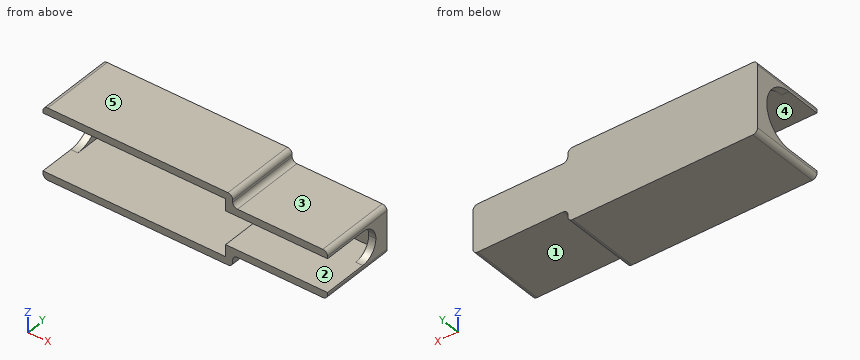
from build123d import *

# Parameters (mm, degrees)
F1_DEPTH = 16
F2_T     = -1.5
F4_DEPTH = 25
F6_DEPTH = 25
F7_R     = 1


with BuildPart() as f1:
    # F0 (on Front) → F1 (new body)
    with BuildSketch(Plane.XZ):
        Polygon((10, 7.5), (-30, 7.5), (-30, -7.5), (10, -7.5), (10, -5), (30, -5), (30, 5), (10, 5), align=None)
    extrude(amount=F1_DEPTH)

    # F2
    f2_openings = [f1.faces().sort_by_distance(p)[0] for p in [
        (-2.5, -16, 0),
    ]]
    offset(amount=F2_T, openings=f2_openings, kind=Kind.INTERSECTION)

    # F3 (on face) → F4 (cut)
    with BuildSketch(Plane.YZ.offset(30)):
        with BuildLine():
            ThreePointArc((-6.5, -3.5), (-10, 0), (-6.5, 3.5))
            Line((-6.5, 3.5), (-16, 3.5))
            Line((-16, 3.5), (-16, -3.5))
            Line((-16, -3.5), (-6.5, -3.5))
        make_face()
        with BuildLine():
            ThreePointArc((-6.5, -3.5), (-4.0251262658, -2.4748737342), (-3, 0))
            ThreePointArc((-3, 0), (-4.0251262658, 2.4748737342), (-6.5, 3.5))
            ThreePointArc((-6.5, 3.5), (-10, 0), (-6.5, -3.5))
        make_face()
    extrude(amount=-F4_DEPTH, mode=Mode.SUBTRACT)

    # F5 (on face) → F6 (cut)
    with BuildSketch(Plane(origin=(-30, 0, 0), x_dir=(0, -1, 0), z_dir=(-1, 0, 0))):
        with BuildLine():
            ThreePointArc((8.5, -6), (12.7426406871, -4.2426406871), (14.5, 0))
            ThreePointArc((14.5, 0), (12.7426406871, 4.2426406871), (8.5, 6))
            ThreePointArc((8.5, 6), (2.5, 0), (8.5, -6))
        make_face()
        with BuildLine():
            ThreePointArc((8.5, 6), (12.7426406871, 4.2426406871), (14.5, 0))
            ThreePointArc((14.5, 0), (12.7426406871, -4.2426406871), (8.5, -6))
            Line((8.5, -6), (16, -6))
            Line((16, -6), (16, 6))
            Line((16, 6), (8.5, 6))
        make_face()
    extrude(amount=-F6_DEPTH, mode=Mode.SUBTRACT)

    # F7
    f7_edges = [f1.edges().sort_by_distance(p)[0] for p in [
        (-30, -8, -7.5),
        (-30, -8, 7.5),
        (10, -8, 5),
        (10, -8, 7.5),
        (10, -8, -7.5),
        (10, -8, -5),
        (30, -8, -5),
        (30, -8, 5),
    ]]
    fillet(f7_edges, radius=F7_R)


solid = f1.part
The model under review builds one solid part; all positions refer to its coordinate system, in mm. Face numbers are marked on the shaded views. A direction names the side the tool comes from. Coordinates: 2 decimals unless noted, no trailing zeros. Order: outer loops, then holes, each group sorted by start corner. A loop starts at its lowest first (then second) coordinate and runs counter-clockwise, first axis right, second up. Notation, with made-up numbers: (7.5, 79.25) -> (50.5, 79.25) arc R22 ccw to (50.5, 115.25) -> close; hole circle Ø10 at (81.5, 3.25). An arc over 180 degrees is marked (long way). Answer in a Markdown table with one row per item.
(1) Consider section B-B (x = -18). Write out the cut boundary in (y, z), plus the area to 3 significant figures.
Answers:
| item | result |
|---|---|
| outline | (-16, -7.5) -> (0, -7.5) -> (0, 7.5) -> (-16, 7.5) -> (-16, 6) -> (-1.5, 6) -> (-1.5, -6) -> (-16, -6) -> close |
| area | 66.0 mm² |
(2) Wall thickness on line 1 along Z through (x, y) = (-11, -9); line 2 along Z through (x, y) = (13, -11.75); line 3 along Y through (x, z) = (-16, 2.25): over which ranges is each line inside the solid? List them lowest first.
Answers:
| item | result |
|---|---|
| line 1 | -7.5 to -6, 6 to 7.5 |
| line 2 | -5 to -3.5, 3.5 to 5 |
| line 3 | -1.5 to 0 |
(3) Consider section D-D (x = 19). Write out the cut boundary in (y, z).
Answers:
| item | result |
|---|---|
| outline | (-16, -5) -> (0, -5) -> (0, 5) -> (-16, 5) -> (-16, 3.5) -> (-1.5, 3.5) -> (-1.5, -3.5) -> (-16, -3.5) -> close |
(4) Machinability: for the marked faces 4 and 5, which of the approach directions +Z, -Z, +X, -X, +Y, -Y give a long, thin tool a straight path to every point of the face, cutting with its end or side? Answer none if there is none.
Answers:
| item | result |
|---|---|
| face 4 | -Y |
| face 5 | +Z, +X, -X, +Y, -Y |
(5) Consider section A-A (y = -11.5). Write out the cut boundary in (x, z), plus the area to 3 significant figures.
Answers:
| item | result |
|---|---|
| outline | (-30, -6.5) arc R1 ccw to (-29, -7.5) -> (9, -7.5) arc R1 ccw to (10, -6.5) -> (10, -6) arc R1 cw to (11, -5) -> (29, -5) arc R1 ccw to (30, -4) -> (30, -3.5) -> (8.5, -3.5) -> (8.5, -6) -> (-30, -6) -> close; (-30, 6) -> (8.5, 6) -> (8.5, 3.5) -> (30, 3.5) -> (30, 4) arc R1 ccw to (29, 5) -> (11, 5) arc R1 cw to (10, 6) -> (10, 6.5) arc R1 ccw to (9, 7.5) -> (-29, 7.5) arc R1 ccw to (-30, 6.5) -> close |
| area | 187 mm² |
(6) Insertion check: pin 1 (3 mm diameter, centred on x = 19, y = -14, fed in from +Z); pin 2 (3.5 mm diameter, centred on x = 7, z = 1, fed in from -Y); pin 3 (5 mm diameter, centred on x = 18, y = -11.5, fed in from -Z). Each pin has a flat end and moves straight along its axis. Give the tip position at first contact, or say it passes through.
Answers:
| item | result |
|---|---|
| pin 1 | z = 5 |
| pin 2 | y = -1.5 |
| pin 3 | z = -5 |
(7) The part is to be moulded in two halves that separate along Z. For the marked faces 1, 2 and 3, say which applies: +Z half, -Z half, draft (parallel to the pull), parting line (faces both ways), or undercut.
Answers:
| item | result |
|---|---|
| face 1 | -Z half |
| face 2 | undercut |
| face 3 | +Z half |
